Can you work these out from the model? Positions are in its coordinate system, mm. Face numbers are marked on the shaded views. A direction names the side the tool comes from. Coordinates: 2 decimals unless noted, no trailing zeros. Loops run counter-clockwise (first coordinate to the right, second up) from the corner with the lowest first, then second, coordinate; pieces in that order, holes last.
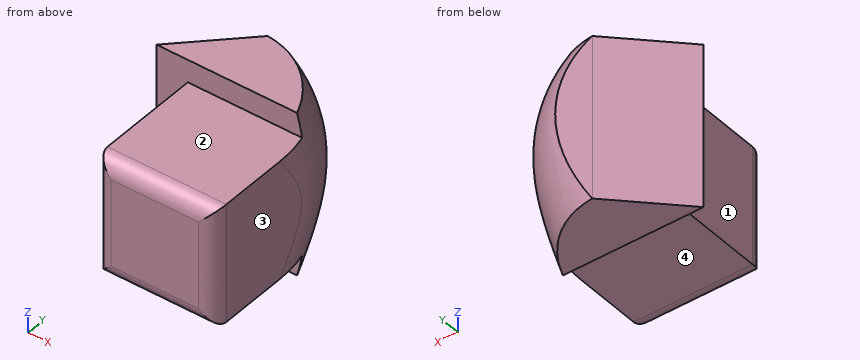
Autodesk Inventor part; units mm, degrees
ref_plane "YZ Plane" through (0, 0, 0) normal (1, 0, 0) x (0, 1, 0)
ref_plane "XZ Plane" through (0, 0, 0) normal (0, 1, 0) x (-1, 0, 0)
ref_plane "XY Plane" through (0, 0, 0) normal (0, 0, 1) x (1, 0, 0)
sketch "Эскиз1" plane through (0, 0, 0) normal (0, 1, 0) x (-1, 0, 0)
  line L0 (1.9, 1.9) -> (-1.9, 1.9)
  line L1 (-1.9, 1.9) -> (-1.9, -1.9)
  line L2 (-1.9, -1.9) -> (1.9, -1.9)
  line L3 (1.9, -1.9) -> (1.9, 1.9)
  line L4 (2.66, 0) -> (-2.66, 0)
  line L5 (0, -2.66) -> (0, 2.66)
  point P0 (0, 0)
  dimension "d0" = 3.8
extrude "Выдавливание1" add sketch "Эскиз1" along normal blind 3.8
sketch "Эскиз2" plane through (0, 3.8, 0) normal (0, 1, 0) x (1, 0, 0)
  line L0 (-2.9, -2.625) -> (1.9, -2.625)
  line L1 (1.9, -2.625) -> (1.9, 2.625)
  line L2 (1.9, 2.625) -> (-2.9, 2.625)
  line L3 (-2.9, 2.625) -> (-2.9, -2.625)
  line L4 (1.9, -1.9) -> (1.9, 1.9)
  line L5 (-3.86, 0) -> (2.86, 0)
  point P0 (0, 0)
  dimension "d3" = 5.25
  dimension "d4" = 4.8
extrude "Выдавливание2" add sketch "Эскиз2" along normal blind 2
sketch "Эскиз5" plane through (1.9, 0, 1.9) normal (1, 0, 0) x (0, 0, -1)
  line L0 (4.525, 3.8) -> (4.525, 5.8)
  line L1 (-0.725, 5.8) -> (4.525, 5.8)
  line L2 (4.525, 5.8) -> (-0.725, 5.8)
  line L3 (-0.725, 3.8) -> (-0.725, 5.8)
  arc A0 (4.525, 5.8) -> (-0.725, 5.8) centre (1.9, 0.9668) ccw
  point P0 (1.9, 0)
  dimension "d10" = 5.5
chamfer "Фаска1" distance 2 angle 45 1 edges at (-2.9, 5.8, 0)
extrude "Выдавливание3" add sketch "Эскиз5" against normal up to surface surface through (-1.9, 4.8, -1.3125) normal (-0.7071068, 0.7071068, 0)
fillet "Сопряжение1" radius 3 1 edges at (1.9, 6.4668, 0)
fillet "Сопряжение2" radius 0.5 4 edges at (1.9, 0, 0) (0, 0, 1.9) (0, 0, -1.9) (-1.9, 0, 0)
properties part number "BUTTON_OUTSIDE"
Item 1: On a 3-axis mill with a long thin cutter (end or side, diameter ignored), from which of +Z, -Z, +X, -X, +Y, -Y can I reach the whole of each face in a straight line? I mean the marked faces 1, 2, 3 and 4. Say none if no direction works.
Results are:
face 1: +Z, -Z, -X, -Y
face 2: +Z, +X, -X, -Y
face 3: +Z, -Z, +X, +Y, -Y
face 4: -Z, +X, -X, -Y
Item 2: Suppose I cut it at A-A, the plane x = -1.1. Please give me the cut outline in (y, z) (3 decimals).
Results are:
outline: (0, -1.4) arc R0.5 ccw to (0.5, -1.9) - (3.8, -1.9) - (3.8, -2.625) - (5.6, -2.625) - (5.6, 2.625) - (3.8, 2.625) - (3.8, 1.9) - (0.5, 1.9) arc R0.5 ccw to (0, 1.4) - close
Item 3: Suppose I cut it at B-B, the plane y = 1. Please give me the cut outline in (x, z).
Results are:
outline: (-1.9, -1.9) - (1.9, -1.9) - (1.9, 1.9) - (-1.9, 1.9) - close
Item 4: I'm going to push flat-ended pins straight in: P1, Ø1, axis at x = -2, z = -1, coming from the -Y side; P2, Ø1.7, axis at x = 1, y = 2, coming from the +Z side; P3, Ø1.5, axis at y = 2, z = 1, coming from the -X side. Where does each tip first touch, or does it pass through?
Results are:
P1: stops at y = 0.01
P2: stops at z = 1.9
P3: stops at x = -1.9
Item 5: I need wall thicknesses on line 1 along Z through (x, y) = (-1.25, 1); line 2 along Y through (x, z) = (-0.9, 2.3). Which ranges of each line are inside material? Lowest first, please.
Results are:
line 1: z = -1.9 to 1.9
line 2: y = 3.8 to 5.8
